```python
from build123d import *

# Parameters (mm, degrees)
BOSS_EXTRUDE1_DEPTH = 1.5
FILLET1_R           = 0.5
SKETCH2_R           = 1.125
CUT_EXTRUDE1_DEPTH  = 26.104780421


with BuildPart() as part:
    # Sketch1 → Boss-Extrude1 (new body)
    with BuildSketch(Plane(origin=(0, 0, 0), x_dir=(1, 0, 0), z_dir=(0, 1, 0))):
        with BuildLine():
            ThreePointArc((7.5, -10), (10, -7.5), (12.5, -10))
            Line((12.5, -10), (20, -10))
            Line((20, -10), (20, -2))
            ThreePointArc((20, -2), (22, 0), (20, 2))
            Line((20, 2), (20, 10))
            Line((20, 10), (12.5, 10))
            ThreePointArc((12.5, 10), (10, 7.5), (7.5, 10))
            Line((7.5, 10), (-8, 10))
            ThreePointArc((-8, 10), (-10, 12), (-12, 10))
            Line((-12, 10), (-20, 10))
            Line((-20, 10), (-20, -10))
            Line((-20, -10), (-12, -10))
            ThreePointArc((-12, -10), (-10, -12), (-8, -10))
            Line((-8, -10), (7.5, -10))
        make_face()
    extrude(amount=BOSS_EXTRUDE1_DEPTH)

    # Fillet1
    fillet1_edges = [part.edges().sort_by_distance(p)[0] for p in [
        (-8, 0.75, 10),
        (-12, 0.75, 10),
        (-20, 0.75, 10),
        (-20, 0.75, -10),
        (-12, 0.75, -10),
        (-8, 0.75, -10),
        (7.5, 0.75, -10),
        (12.5, 0.75, -10),
        (20, 0.75, -10),
        (20, 0.75, -2),
        (20, 0.75, 2),
        (20, 0.75, 10),
        (12.5, 0.75, 10),
        (7.5, 0.75, 10),
    ]]
    fillet(fillet1_edges, radius=FILLET1_R)

    # Sketch2 → Cut-Extrude1 (cut, through all)
    with BuildSketch(Plane(origin=(0, 1.5, 0), x_dir=(1, 0, 0), z_dir=(0, 1, 0))):
        with Locations(Location((20, 0, 0), (0, 0, 270))):
            Circle(SKETCH2_R)
        with Locations(Location((-10, -10, 0), (0, 0, 270))):
            Circle(SKETCH2_R)
        with Locations(Location((-10, 10, 0), (0, 0, 270))):
            Circle(SKETCH2_R)
    extrude(amount=-CUT_EXTRUDE1_DEPTH, mode=Mode.SUBTRACT)


solid = part.part
```
Geometry: final body of the model. Coordinates: model frame, mm. A direction names the side the tool comes from. Coordinates: 2 decimals unless noted, no trailing zeros. Order: outer loops, then holes, each group sorted by start corner. A loop starts at its lowest first (then second) coordinate and runs counter-clockwise, first axis right, second up. Notation, with made-up numbers: M 34,74 L 71,74 A16 cw 71,102 Z; hole C -29,16 d9. An arc over 180 degrees is marked long. Answer as CSV lines item,"result".
Q1. Section D-D on z = -6.5. Return the cut outline in (x, y).
Answers:
outline,"M -20,0 L 20,0 L 20,1.5 L -20,1.5 Z"
Q2. Set-up query: faces 5 (the flat face through (-16, 1, -10)), 6 (the flat face through (16, 1, 10)), 7 (the flat face through (16, 1, -10)), 8 (the flat face through (-16, 1, 10)). Return all of +Z, -Z, +X, -X, +Y, -Y with unobstructed straight access to the full face (end or side cutting, diameter ignored); none if empty.
Answers:
face 5,"-Z, -X, +Y, -Y"
face 6,"+Z, +X, +Y, -Y"
face 7,"-Z, +X, +Y, -Y"
face 8,"+Z, -X, +Y, -Y"
Q3. Section A-A on z = 0. Return the cut outline in (x, y) (3 decimals), and give its area (3 significant figures).
Answers:
outline,"M -20,0 L 18.875,0 L 18.875,1.5 L -20,1.5 Z; M 21.125,0 L 22,0 L 22,1.5 L 21.125,1.5 Z"
area,"59.6 mm^2"
Q4. Line query: probe 1 along X at (y, z) = (0.4, -4.25); probe 2 along Z at (x, y) = (2.5, 0.3); probe 3 along X at (y, z) = (0.85, 8.5). Output: solid intervals per line, ascending. Write a range as [from, to].
Answers:
probe 1,"x = [-20, 20]"
probe 2,"z = [-10, 10]"
probe 3,"x = [-20, 8], [12, 20]"
Q5. Draft query along X for faces 1 (the flat face through (0, 1, 10)), 2 (the cylindrical face through (-10.998, 0.76, -9.481)), 3 (the cylindrical face through (-10, 1, 12)), 4 (the flat face through (20, 1, 6)). Return one class per face: pulls with the +X half, pulls with the -X half, needs draft (parallel to the pull), parting line crosses it, or undercut.
Answers:
face 1,"needs draft"
face 2,"undercut"
face 3,"parting line crosses it"
face 4,"pulls with the +X half"
Q6. First-contact query: P1, Ø1.5, axis at x = -6.5, z = -5.5, coming from the -Y side; P2, Ø0.8, axis at y = 0.5, z = 6, coming from the +X side; P3, Ø0.8, axis at x = -15, y = 0.5, coming from the +Z side. Flat tips, straight axial feed; report the tip coordinate or a pass-through.
Answers:
P1,"stops at y = 0"
P2,"stops at x = 20"
P3,"stops at z = 10"
Q7. Section B-B on y = 1.25. Count the separate pieces of the cut face and the enclosed holes in it, and give its area (3 significant figures).
Answers:
separate pieces,"1"
enclosed holes,"3"
area,"787 mm^2"
Q8. Section C-C on x = -10. Return the cut outline in (y, z) (3 decimals), and give its area (4 significant figures).
Answers:
outline,"M 0,-12 L 1.5,-12 L 1.5,-11.125 L 0,-11.125 Z; M 0,-8.875 L 1.5,-8.875 L 1.5,8.875 L 0,8.875 Z; M 0,11.125 L 1.5,11.125 L 1.5,12 L 0,12 Z"
area,"29.25 mm^2"
